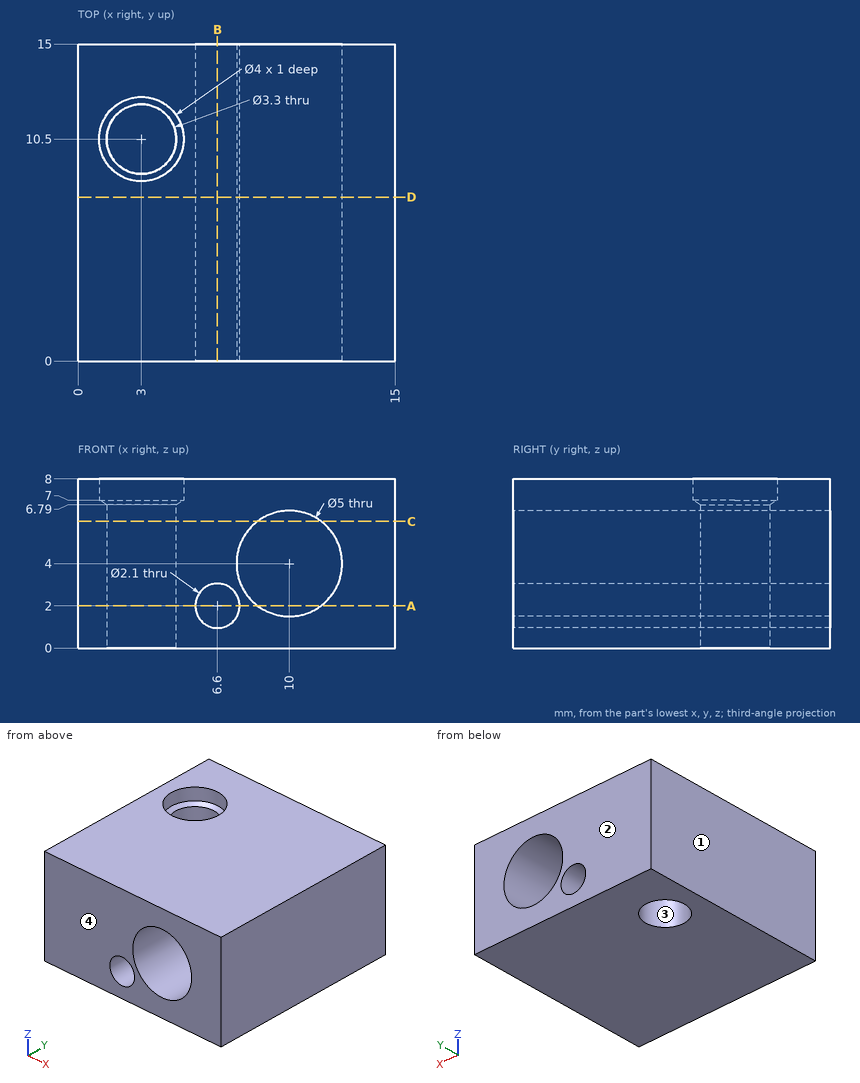
Verification items for this drawing (mm, ordinates from the low corner). Round coordinates to 2 decimals unless told otherwise and drop trailing zeros. Order: outer loops, then holes, each group sorted by start corner. A loop starts at its lowest first (then second) coordinate and runs counter-clockwise, first axis right, second up.
1) Material ranges on line 1 (Z direction, x = 6.6, y = 3.5); line 2 (Z direction, x = 10, y = 7.25); line 3 (Y direction, x = 3, z = 7.35), recorded low to high.
Geometry says:
line 1: z = 0 to 0.95, 3.05 to 8
line 2: z = 0 to 1.5, 6.5 to 8
line 3: y = 0 to 8.5, 12.5 to 15
2) Cross-section at D-D, the plane y = 7.75. Record the cut outline in (x, z).
Geometry says:
outline: (0, 0) - (15, 0) - (15, 8) - (0, 8) - close; hole circle Ø2.1 at (6.6, 2); hole circle Ø5 at (10, 4)
3) Cross-section at A-A, the plane z = 2. Record the cut outline in (x, y).
Geometry says:
outline: (0, 0) - (5.55, 0) - (5.55, 15) - (0, 15) - close; (7.65, 0) - (8.5, 0) - (8.5, 15) - (7.65, 15) - close; (11.5, 0) - (15, 0) - (15, 15) - (11.5, 15) - close; hole circle Ø3.3 at (3, 10.5)
4) Draft check along Y on the marked faces 1, 2, 3 and 4. Enter one of: +Y half, -Y half, draft (parallel to the pull), parting line (faces both ways), or undercut.
Geometry says:
face 1: draft
face 2: +Y half
face 3: undercut
face 4: -Y half
5) Cross-section at B-B, the plane x = 6.6. Record the cut outline in (y, z), plus the area to 3 significant figures.
Geometry says:
outline: (0, 0) - (15, 0) - (15, 0.95) - (0, 0.95) - close; (0, 3.05) - (15, 3.05) - (15, 8) - (0, 8) - close
area: 88.5 mm2
6) Depth check by flat-ended pin: pin 1 (2.5 mm diameter, centred on x = 6.6, z = 2, fed in from +Y). Enter the tip coordinate at first touch or a pass-through.
Geometry says:
pin 1: stops at y = 15
7) Cross-section at C-C, the plane z = 6. Record the cut outline in (x, y).
Geometry says:
outline: (0, 0) - (8.5, 0) - (8.5, 15) - (0, 15) - close; (11.5, 0) - (15, 0) - (15, 15) - (11.5, 15) - close; hole circle Ø3.3 at (3, 10.5)
